from build123d import *

# Parameters (mm, degrees)
BASE_DEPTH              = 2
SKETCH2_W               = 3
SKETCH2_H               = 40
SERVOLEG_DEPTH          = 18.6
SKETCH3_R               = 1.3
SERVOCUTOUT_DEPTH       = 80.942955098
FILLET2_R               = 10
FILLET3_R               = 2
FILLET4_R               = 5
SKETCH4_R               = 1.5
MATERIALREMOVAL_DEPTH   = 102.88839318
MOUNTINGHOLES_OUTLINE_R = 1.5
MOUNTINGHOLES_DEPTH     = 2
FIXTOPRINT3D_DEPTH      = 0.2


# Read off the part's stored shape, not the designer's step: MountingHoles
with BuildPart() as part:
    # Sketch1 → Base (new body)
    with BuildSketch(Plane(origin=(0, 0, 0), x_dir=(1, 0, 0), z_dir=(0, 1, 0))):
        Polygon((18.863636364, -70.303030303), (1.363636364, -30.303030303), (1.363636364, 29.696969697), (36.363636364, 29.696969697), (36.363636364, -70.303030303), align=None)
    extrude(amount=BASE_DEPTH)

    # Sketch2 → ServoLeg (add)
    with BuildSketch(Plane(origin=(0, 2, 0), x_dir=(1, 0, 0), z_dir=(0, 1, 0))):
        with Locations((2.863636364, 9.696969697)):
            Rectangle(SKETCH2_W, SKETCH2_H)
    extrude(amount=SERVOLEG_DEPTH)

    # Sketch3 → ServoCutout (cut, through all)
    with BuildSketch(Plane(origin=(4.363636364, 0, 0), x_dir=(0, 0, -1), z_dir=(1, 0, 0))):
        with Locations((23.496969697, 14.25)):
            Circle(SKETCH3_R)
        with Locations((-4.103030303, 14.25)):
            Circle(SKETCH3_R)
        Polygon((21.496969697, 20.6), (-2.103030303, 20.6), (-2.103030303, 15.55), (-2.103030303, 12.95), (-2.103030303, 7.9), (21.496969697, 7.9), (21.496969697, 12.95), (21.496969697, 15.55), align=None)
    extrude(amount=-SERVOCUTOUT_DEPTH, mode=Mode.SUBTRACT)

    # Fillet2
    fillet2_edges = [part.edges().sort_by_distance(p)[0] for p in [
        (18.863636364, 1, 70.303030303),
        (1.363636364, 1, 30.303030303),
    ]]
    fillet(fillet2_edges, radius=FILLET2_R)

    # Fillet3
    fillet3_edges = [part.edges().sort_by_distance(p)[0] for p in [
        (2.863636364, 2, 10.303030303),
        (4.363636364, 2, -9.696969697),
    ]]
    fillet(fillet3_edges, radius=FILLET3_R)

    # Fillet4
    fillet4_edges = [part.edges().sort_by_distance(p)[0] for p in [
        (2.863636364, 20.6, 10.303030303),
        (2.863636364, 20.6, -29.696969697),
    ]]
    fillet(fillet4_edges, radius=FILLET4_R)

    # Mirror1: part across plane


with BuildPart() as part_1:
    add(part.part)
    add(part.part.mirror(Plane(origin=(36.363636364, 2, -29.696969697), x_dir=(0, 0, 1), z_dir=(-1, 0, 0))))

    # Sketch4 → MaterialRemoval (cut, through all)
    with BuildSketch(Plane(origin=(0, 2, 0), x_dir=(1, 0, 0), z_dir=(0, 1, 0))):
        with Locations(Location((9.363636364, 26.696969697, 0), (0, 0, 270))):
            Circle(SKETCH4_R)
    extrude(amount=-MATERIALREMOVAL_DEPTH, mode=Mode.SUBTRACT)

    # MountingHoles outline → MountingHoles (cut)
    with BuildSketch(Plane(origin=(0, 0, 0), x_dir=(1, 0, 0), z_dir=(0, 1, 0))):
        with Locations((9.363636364, -36.303030303)):
            Circle(MOUNTINGHOLES_OUTLINE_R)
        with Locations((63.363636364, 26.696969697)):
            Circle(MOUNTINGHOLES_OUTLINE_R)
        with Locations((63.363636364, 17.696969697)):
            Circle(MOUNTINGHOLES_OUTLINE_R)
        with Locations((63.363636364, 8.696969697)):
            Circle(MOUNTINGHOLES_OUTLINE_R)
        with Locations((18.363636364, 26.696969697)):
            Circle(MOUNTINGHOLES_OUTLINE_R)
        with Locations((18.363636364, 17.696969697)):
            Circle(MOUNTINGHOLES_OUTLINE_R)
        with Locations((18.363636364, 8.696969697)):
            Circle(MOUNTINGHOLES_OUTLINE_R)
        with Locations((18.363636364, -0.303030303)):
            Circle(MOUNTINGHOLES_OUTLINE_R)
        with Locations((18.363636364, -9.303030303)):
            Circle(MOUNTINGHOLES_OUTLINE_R)
        with Locations((18.363636364, -18.303030303)):
            Circle(MOUNTINGHOLES_OUTLINE_R)
        with Locations((18.363636364, -27.303030303)):
            Circle(MOUNTINGHOLES_OUTLINE_R)
        with Locations((18.363636364, -36.303030303)):
            Circle(MOUNTINGHOLES_OUTLINE_R)
        with Locations((9.363636364, -27.303030303)):
            Circle(MOUNTINGHOLES_OUTLINE_R)
        with Locations((9.363636364, -18.303030303)):
            Circle(MOUNTINGHOLES_OUTLINE_R)
        with Locations((9.363636364, -9.303030303)):
            Circle(MOUNTINGHOLES_OUTLINE_R)
        with Locations((9.363636364, -0.303030303)):
            Circle(MOUNTINGHOLES_OUTLINE_R)
        with Locations((9.363636364, 8.696969697)):
            Circle(MOUNTINGHOLES_OUTLINE_R)
        with Locations((9.363636364, 17.696969697)):
            Circle(MOUNTINGHOLES_OUTLINE_R)
        with Locations((18.363636364, -54.303030303)):
            Circle(MOUNTINGHOLES_OUTLINE_R)
        with Locations((18.363636364, -45.303030303)):
            Circle(MOUNTINGHOLES_OUTLINE_R)
        with Locations((36.363636364, -63.303030303)):
            Circle(MOUNTINGHOLES_OUTLINE_R)
        with Locations((27.363636364, 26.696969697)):
            Circle(MOUNTINGHOLES_OUTLINE_R)
        with Locations((27.363636364, 17.696969697)):
            Circle(MOUNTINGHOLES_OUTLINE_R)
        with Locations((27.363636364, 8.696969697)):
            Circle(MOUNTINGHOLES_OUTLINE_R)
        with Locations((36.363636364, -54.303030303)):
            Circle(MOUNTINGHOLES_OUTLINE_R)
        with Locations((36.363636364, -45.303030303)):
            Circle(MOUNTINGHOLES_OUTLINE_R)
        with Locations((36.363636364, -36.303030303)):
            Circle(MOUNTINGHOLES_OUTLINE_R)
        with Locations((36.363636364, -27.303030303)):
            Circle(MOUNTINGHOLES_OUTLINE_R)
        with Locations((27.363636364, -0.303030303)):
            Circle(MOUNTINGHOLES_OUTLINE_R)
        with Locations((27.363636364, -9.303030303)):
            Circle(MOUNTINGHOLES_OUTLINE_R)
        with Locations((27.363636364, -18.303030303)):
            Circle(MOUNTINGHOLES_OUTLINE_R)
        with Locations((27.363636364, -27.303030303)):
            Circle(MOUNTINGHOLES_OUTLINE_R)
        with Locations((27.363636364, -36.303030303)):
            Circle(MOUNTINGHOLES_OUTLINE_R)
        with Locations((27.363636364, -45.303030303)):
            Circle(MOUNTINGHOLES_OUTLINE_R)
        with Locations((27.363636364, -54.303030303)):
            Circle(MOUNTINGHOLES_OUTLINE_R)
        with Locations((27.363636364, -63.303030303)):
            Circle(MOUNTINGHOLES_OUTLINE_R)
        with Locations((54.363636364, -0.303030303)):
            Circle(MOUNTINGHOLES_OUTLINE_R)
        with Locations((54.363636364, -9.303030303)):
            Circle(MOUNTINGHOLES_OUTLINE_R)
        with Locations((54.363636364, -18.303030303)):
            Circle(MOUNTINGHOLES_OUTLINE_R)
        with Locations((54.363636364, -27.303030303)):
            Circle(MOUNTINGHOLES_OUTLINE_R)
        with Locations((45.363636364, 26.696969697)):
            Circle(MOUNTINGHOLES_OUTLINE_R)
        with Locations((54.363636364, -54.303030303)):
            Circle(MOUNTINGHOLES_OUTLINE_R)
        with Locations((54.363636364, -45.303030303)):
            Circle(MOUNTINGHOLES_OUTLINE_R)
        with Locations((54.363636364, -36.303030303)):
            Circle(MOUNTINGHOLES_OUTLINE_R)
        with Locations((63.363636364, -0.303030303)):
            Circle(MOUNTINGHOLES_OUTLINE_R)
        with Locations((63.363636364, -9.303030303)):
            Circle(MOUNTINGHOLES_OUTLINE_R)
        with Locations((63.363636364, -18.303030303)):
            Circle(MOUNTINGHOLES_OUTLINE_R)
        with Locations((63.363636364, -27.303030303)):
            Circle(MOUNTINGHOLES_OUTLINE_R)
        with Locations((54.363636364, 8.696969697)):
            Circle(MOUNTINGHOLES_OUTLINE_R)
        with Locations((54.363636364, 17.696969697)):
            Circle(MOUNTINGHOLES_OUTLINE_R)
        with Locations((54.363636364, 26.696969697)):
            Circle(MOUNTINGHOLES_OUTLINE_R)
        with Locations((63.363636364, -36.303030303)):
            Circle(MOUNTINGHOLES_OUTLINE_R)
        with Locations((45.363636364, -54.303030303)):
            Circle(MOUNTINGHOLES_OUTLINE_R)
        with Locations((45.363636364, -63.303030303)):
            Circle(MOUNTINGHOLES_OUTLINE_R)
        with Locations((36.363636364, 26.696969697)):
            Circle(MOUNTINGHOLES_OUTLINE_R)
        with Locations((36.363636364, 17.696969697)):
            Circle(MOUNTINGHOLES_OUTLINE_R)
        with Locations((36.363636364, 8.696969697)):
            Circle(MOUNTINGHOLES_OUTLINE_R)
        with Locations((36.363636364, -0.303030303)):
            Circle(MOUNTINGHOLES_OUTLINE_R)
        with Locations((36.363636364, -9.303030303)):
            Circle(MOUNTINGHOLES_OUTLINE_R)
        with Locations((36.363636364, -18.303030303)):
            Circle(MOUNTINGHOLES_OUTLINE_R)
        with Locations((45.363636364, -45.303030303)):
            Circle(MOUNTINGHOLES_OUTLINE_R)
        with Locations((45.363636364, -36.303030303)):
            Circle(MOUNTINGHOLES_OUTLINE_R)
        with Locations((45.363636364, -27.303030303)):
            Circle(MOUNTINGHOLES_OUTLINE_R)
        with Locations((45.363636364, -18.303030303)):
            Circle(MOUNTINGHOLES_OUTLINE_R)
        with Locations((45.363636364, -9.303030303)):
            Circle(MOUNTINGHOLES_OUTLINE_R)
        with Locations((45.363636364, -0.303030303)):
            Circle(MOUNTINGHOLES_OUTLINE_R)
        with Locations((45.363636364, 8.696969697)):
            Circle(MOUNTINGHOLES_OUTLINE_R)
        with Locations((45.363636364, 17.696969697)):
            Circle(MOUNTINGHOLES_OUTLINE_R)
    extrude(amount=MOUNTINGHOLES_DEPTH, mode=Mode.SUBTRACT)

    # Sketch5 → FixToPrint3d (add)
    with BuildSketch(Plane.XZ):
        with BuildLine():
            Line((47.323480616, 70.303030303), (25.403792111, 70.303030303))
            ThreePointArc((25.403792111, 70.303030303), (19.930305261, 68.672076945), (16.242218762, 64.311218643))
            Line((16.242218762, 64.311218643), (2.202063015, 32.219434077))
            ThreePointArc((2.202063015, 32.219434077), (1.575487062, 30.258715701), (1.363636364, 28.211245736))
            Line((1.363636364, 28.211245736), (1.363636364, -29.696969697))
            Line((1.363636364, -29.696969697), (71.363636364, -29.696969697))
            Line((71.363636364, -29.696969697), (71.363636364, 28.211245736))
            ThreePointArc((71.363636364, 28.211245736), (71.151785665, 30.258715701), (70.525209713, 32.219434077))
            Line((70.525209713, 32.219434077), (56.485053965, 64.311218643))
            ThreePointArc((56.485053965, 64.311218643), (52.796967466, 68.672076945), (47.323480616, 70.303030303))
        make_face()
    extrude(amount=FIXTOPRINT3D_DEPTH)


solid = part_1.part
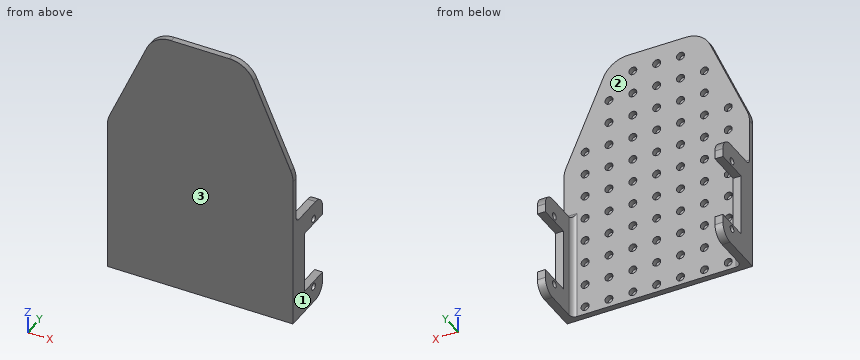
The listing builds one solid part. Answer for the finished solid, in the listing's coordinates (mm). Face numbers are marked on the shaded views. Coordinates: 2 decimals unless noted, no trailing zeros. Loops run counter-clockwise (first coordinate to the right, second up) from the corner with the lowest first, then second, coordinate; pieces in that order, holes last.
1) Find section C-C on x = 31. Write down the section's boundary in (y, z).
2) Find section B-B on y = 9.75. Write down the section's boundary in (x, z).
3) Flat-ended cylindrical pins translate along their axes: pin 1 Ø2.5 at (x, z) = (18.36, 18.3) entering from +Y; pin 2 Ø3.5 at (x, z) = (36, 36) entering from +Y; pin 3 Ø10 at (y, z) = (6.5, 54) entering from +X; pin 4 Ø4 at (y, z) = (7, 12.5) entering from -X. Find the tip coordinate at first contact, or state that the pin passes through.
4) Find section A-A on y = 14.25. Give the number of separate pieces and of enclosed holes in the cut face, then the cut area to 3 significant figures.
5) Determine the mould class of the marked faces 1, 2 and 3 for opening direction X: pulls with the +X half, pulls with the -X half, needs draft (parallel to the pull), parting line crosses it, or undercut.
6) Find the intervals of material crossed by L1, parallel to X at y = 16.75, z = 10; L2, parallel to Y at x = 44.5, z = 58; L3, parallel to Y at x = 45.5, z = 54.5, in increasing order.
Values:
1. outline: (-0.2, -29.7) - (2, -29.7) - (2, 70.3) - (-0.2, 70.3) - close
2. outline: (1.36, -29.7) - (4.36, -29.7) - (4.36, -21.5) - (1.36, -21.5) - close; (1.36, 2.1) - (4.36, 2.1) - (4.36, 10.3) - (1.36, 10.3) - close; (68.36, -29.7) - (71.36, -29.7) - (71.36, -21.5) - (68.36, -21.5) - close; (68.36, 2.1) - (71.36, 2.1) - (71.36, 10.3) - (68.36, 10.3) - close
3. pin 1: stops at y = 0
3. pin 2: stops at y = 2
3. pin 3: stops at x = 61.95
3. pin 4: passes through
4. separate pieces: 8
4. enclosed holes: 0
4. area: 67.2 mm2
5. face 1: pulls with the +X half
5. face 2: undercut
5. face 3: needs draft
6. L1: x = 1.36 to 4.36, 68.36 to 71.36
6. L2: y = -0.2 to 2
6. L3: y = -0.2 to 0
